from build123d import *

# Parameters (mm, degrees)
SKETCH_W        = 94
SKETCH_H        = 83
PAD_DEPTH       = 38
POCKET_DEPTH    = 34
SKETCH002_R     = 6
PAD001_DEPTH    = 5
SKETCH004_W     = 13
SKETCH004_H     = 12
SKETCH004_W_2   = 10
POCKET001_DEPTH = 5
SKETCH005_R     = 1.9
POCKET002_DEPTH = 9.001
POCKET003_DEPTH = 4
SKETCH007_R     = 2.25
POCKET004_DEPTH = 38.001
POCKET005_DEPTH = 4
FILLET_R        = 3
FILLET001_R     = 3
FILLET002_R     = 3
FILLET003_R     = 3


with BuildPart() as part:
    # Sketch → Pad (new body)
    with BuildSketch(Plane.XY):
        Rectangle(SKETCH_W, SKETCH_H)
    extrude(amount=PAD_DEPTH)

    # Sketch001 (on Face6 of Pad) → Pocket (cut)
    with BuildSketch(Plane.XY.offset(38)):
        with BuildLine():
            Line((-37, 37.5), (37, 37.5))
            ThreePointArc((37, 37.5), (38.757359, 33.257359), (43, 31.5))
            Line((43, 31.5), (43, -31.5))
            ThreePointArc((43, -31.5), (38.757359, -33.257359), (37, -37.5))
            Line((37, -37.5), (-37, -37.5))
            ThreePointArc((-37, -37.5), (-38.757359, -33.257359), (-43, -31.5))
            Line((-43, -31.5), (-43, 31.5))
            ThreePointArc((-43, 31.5), (-38.757359, 33.257359), (-37, 37.5))
        make_face()
    extrude(amount=-POCKET_DEPTH, mode=Mode.SUBTRACT)

    # Sketch002 (on Face15 of Pocket) → Pad001 (join)
    with BuildSketch(Plane.XY.offset(4)):
        with Locations((-23.3, 22.5)):
            Circle(SKETCH002_R)
        with Locations((24.5, 21.4)):
            Circle(SKETCH002_R)
        with Locations((-18.6, -29.4)):
            Circle(SKETCH002_R)
        with Locations((9.3, -29.4)):
            Circle(SKETCH002_R)
    extrude(amount=PAD001_DEPTH)

    # Sketch004 → Pocket001 (cut)
    with BuildSketch(Plane(origin=(0, 41.5, 0), x_dir=(-1, 0, 0), z_dir=(0, 1, 0))):
        with Locations((-11.5, 18)):
            Rectangle(SKETCH004_W, SKETCH004_H)
        with Locations((18, 18)):
            Rectangle(SKETCH004_W_2, SKETCH004_H)
    extrude(amount=-POCKET001_DEPTH, mode=Mode.SUBTRACT)

    # Sketch005 (on Face30 of Pocket001) → Pocket002 (cut, through all)
    with BuildSketch(Plane.XY.offset(9)):
        with Locations((-23.3, 22.5)):
            Circle(SKETCH005_R)
        with Locations((24.5, 21.4)):
            Circle(SKETCH005_R)
        with Locations((-18.6, -29.4)):
            Circle(SKETCH005_R)
        with Locations((9.3, -29.4)):
            Circle(SKETCH005_R)
    extrude(amount=-POCKET002_DEPTH, mode=Mode.SUBTRACT)

    # Sketch006 (on Face3 of Pocket002) → Pocket003 (cut)
    with BuildSketch(Plane(origin=(0, 0, 0), x_dir=(1, 0, 0), z_dir=(0, 0, -1))):
        Polygon((-15.75, 27.754552), (-15.75, 31.045448), (-18.6, 32.690897), (-21.45, 31.045448), (-21.45, 27.754552), (-18.6, 26.109103), align=None)
        Polygon((12.15, 27.754552), (12.15, 31.045448), (9.3, 32.690897), (6.45, 31.045448), (6.45, 27.754552), (9.3, 26.109103), align=None)
        Polygon((-20.45, -24.145448), (-20.45, -20.854552), (-23.3, -19.209103), (-26.15, -20.854552), (-26.15, -24.145448), (-23.3, -25.790897), align=None)
        Polygon((27.35, -23.045448), (27.35, -19.754552), (24.5, -18.109103), (21.65, -19.754552), (21.65, -23.045448), (24.5, -24.690897), align=None)
    extrude(amount=-POCKET003_DEPTH, mode=Mode.SUBTRACT)

    # Sketch007 (on Face4 of Pocket003) → Pocket004 (cut, through all)
    with BuildSketch(Plane.XY.offset(38)):
        with Locations((-43, 37.5)):
            Circle(SKETCH007_R)
        with Locations((43, 37.5)):
            Circle(SKETCH007_R)
        with Locations((43, -37.5)):
            Circle(SKETCH007_R)
        with Locations((-43, -37.5)):
            Circle(SKETCH007_R)
    extrude(amount=-POCKET004_DEPTH, mode=Mode.SUBTRACT)

    # Sketch008 (on Face3 of Pocket004) → Pocket005 (cut)
    with BuildSketch(Plane(origin=(0, 0, 0), x_dir=(1, 0, 0), z_dir=(0, 0, -1))):
        Polygon((-43, -41.830127), (-39.25, -39.665064), (-39.25, -35.334936), (-43, -33.169873), (-46.75, -35.334936), (-46.75, -39.665064), align=None)
        Polygon((43, -41.830127), (46.75, -39.665064), (46.75, -35.334936), (43, -33.169873), (39.25, -35.334936), (39.25, -39.665064), align=None)
        Polygon((-39.25, 35.334936), (-39.25, 39.665064), (-43, 41.830127), (-46.75, 39.665064), (-46.75, 35.334936), (-43, 33.169873), align=None)
        Polygon((43, 33.169873), (46.75, 35.334936), (46.75, 39.665064), (43, 41.830127), (39.25, 39.665064), (39.25, 35.334936), align=None)
    extrude(amount=-POCKET005_DEPTH, mode=Mode.SUBTRACT)

    # Fillet
    fillet_edges = [part.edges().sort_by_distance(p)[0] for p in [
        (-47, 41.5, 19),
    ]]
    fillet(fillet_edges, radius=FILLET_R)

    # Fillet001
    fillet001_edges = [part.edges().sort_by_distance(p)[0] for p in [
        (-47, -41.5, 19),
    ]]
    fillet(fillet001_edges, radius=FILLET001_R)

    # Fillet002
    fillet002_edges = [part.edges().sort_by_distance(p)[0] for p in [
        (47, -41.5, 19),
    ]]
    fillet(fillet002_edges, radius=FILLET002_R)

    # Fillet003
    fillet003_edges = [part.edges().sort_by_distance(p)[0] for p in [
        (47, 41.5, 19),
    ]]
    fillet(fillet003_edges, radius=FILLET003_R)


solid = part.part
Verification items for the finished model (mm, model axes). A direction names the side the tool comes from. Coordinates: 2 decimals unless noted, no trailing zeros. Order: outer loops, then holes, each group sorted by start corner. A loop starts at its lowest first (then second) coordinate and runs counter-clockwise, first axis right, second up. Notation, with made-up numbers: (3.5, -24) -> (61.5, -24) arc R32 ccw to (61.5, 12) -> close; hole circle Ø3 at (3.5, -38). An arc over 180 degrees is marked (long way). Use CSV: the item, a comma, the result in double quotes. Start each with the question number.
Q1. Depth check by flat-ended pin: P1, Ø3, axis at x = -18.6, y = -29.4, coming from the +Z side; P2, Ø1.7, axis at x = -22, y = 23, coming from the -Z side; P3, Ø5, axis at x = 15.5, y = 20, coming from the +Z side. Enter the tip coordinate at first touch or a pass-through.
Q2. Section check D-D, the plane y = 0.5. Record the cut outline in (x, z).
Q3. Section check B-B, the plane z = 27. Record the cut outline in (x, y).
Q4. Thickness scan on line 1 along Y through (x, z) = (15.5, 26); line 2 along X through (y, z) = (-5.5, 7); line 3 along X through (y, z) = (-38, 9.5). Record the ranges inside material, lowest first.
Q5. Section check C-C, the plane x = -9.5. Record the cut outline in (y, z).
Q6. Draft check along Z on faces 5 (the flat face through (40.82, 40.57, 1.97)), 6 (the flat face through (5, 40, 18)), 7 (the flat face through (-1, 1, 0)). Enter one of: +Z half, -Z half, draft (parallel to the pull), parting line (faces both ways), or undercut.
Q7. Section check A-A, the plane z = 14. Record the cut outline in (x, y), and give its area (3 significant figures).
Q8. Tool access check on faces 1 (the cylindrical face through (46.1, -40.64, 19.27)), 2 (the flat face through (39.25, 37, 2)), 3 (the flat face through (-18, 40, 24)), 4 (the cylindrical face through (19.74, 17.75, 6.46)). Record the directions out of +Z, -Z, +X, -X, +Y, -Y that give a thin tool (end or side, any length) a straight path to the whole face; none if there is none.
Returned:
1,P1,"passes through"
1,P2,"stops at z = 4"
1,P3,"stops at z = 4"
2,outline,"(-47, 0) -> (47, 0) -> (47, 38) -> (43, 38) -> (43, 4) -> (-43, 4) -> (-43, 38) -> (-47, 38) -> close"
3,outline,"(-47, -38.5) arc R3 ccw to (-44, -41.5) -> (44, -41.5) arc R3 ccw to (47, -38.5) -> (47, 38.5) arc R3 ccw to (44, 41.5) -> (-44, 41.5) arc R3 ccw to (-47, 38.5) -> close; hole circle Ø4.5 at (-43, -37.5); hole circle Ø4.5 at (-43, 37.5); hole (-43, -31.5) arc R6 cw to (-37, -37.5) -> (37, -37.5) arc R6 cw to (43, -31.5) -> (43, 31.5) arc R6 cw to (37, 37.5) -> (-37, 37.5) arc R6 cw to (-43, 31.5) -> close; hole circle Ø4.5 at (43, -37.5); hole circle Ø4.5 at (43, 37.5)"
4,line 1,"y = -41.5 to -37.5, 37.5 to 41.5"
4,line 2,"x = -47 to -43, 43 to 47"
4,line 3,"x = -47 to -45.19, -40.81 to 40.81, 45.19 to 47"
5,outline,"(-41.5, 0) -> (41.5, 0) -> (41.5, 38) -> (37.5, 38) -> (37.5, 4) -> (-37.5, 4) -> (-37.5, 38) -> (-41.5, 38) -> close"
6,face 5,"draft"
6,face 6,"undercut"
6,face 7,"-Z half"
7,outline,"(-47, -38.5) arc R3 ccw to (-44, -41.5) -> (44, -41.5) arc R3 ccw to (47, -38.5) -> (47, 38.5) arc R3 ccw to (44, 41.5) -> (18, 41.5) -> (18, 37.5) -> (37, 37.5) arc R6 ccw to (43, 31.5) -> (43, -31.5) arc R6 ccw to (37, -37.5) -> (-37, -37.5) arc R6 ccw to (-43, -31.5) -> (-43, 31.5) arc R6 ccw to (-37, 37.5) -> (-23, 37.5) -> (-23, 41.5) -> (-44, 41.5) arc R3 ccw to (-47, 38.5) -> close; (-13, 37.5) -> (5, 37.5) -> (5, 41.5) -> (-13, 41.5) -> close; hole circle Ø4.5 at (-43, -37.5); hole circle Ø4.5 at (-43, 37.5); hole circle Ø4.5 at (43, -37.5); hole circle Ø4.5 at (43, 37.5)"
7,area,"1,300 mm^2"
8,face 1,"+Z, -Z, +X, -Y"
8,face 2,"-Z"
8,face 3,"+Y"
8,face 4,"+Z"
